Here's the drawing with two shaded views (mm, measured from the low corner). I have some questions. Coordinates: 2 decimals unless noted, no trailing zeros. Order: outer loops, then holes, each group sorted by start corner. A loop starts at its lowest first (then second) coordinate and runs counter-clockwise, first axis right, second up. Notation, with made-up numbers: (-40, 61.5) - (-31, 61.5) arc R16 ccw to (-31, 73.5) - close; hole circle Ø3 at (-16, 20.5). An arc over 180 degrees is marked (long way). One line per item, written item: value. Start each with the question number.
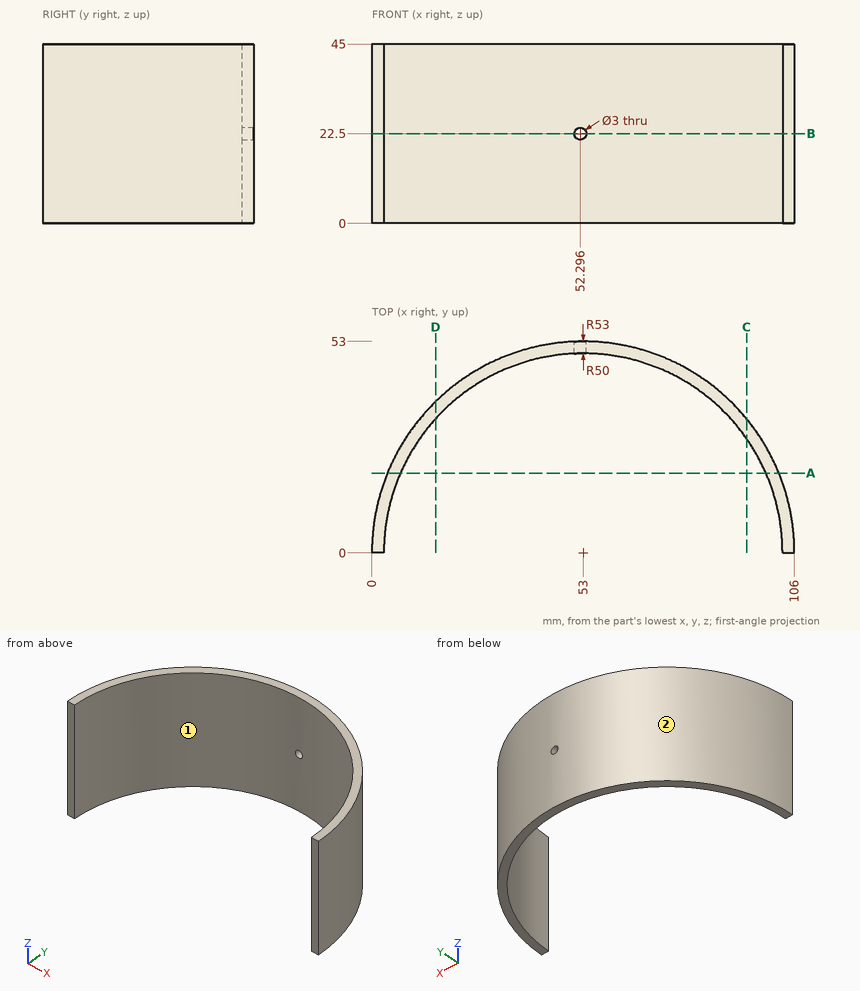
Q1. I want a section at A-A on y = 20. Please give me the cut outline in (x, z) (1 decimal).
Q2. If I drill on L1, parallel to X at y = 21.5, z = 7.5 (1 decimal); L2, parallel to X at y = 9, z = 41; L3, parallel to Y at x = 52, z = 36, over which ranges is the centre line in solid material (lowest first)?
Q3. We'd pull the mould along X, two halves only. Please class the marked faces 1 and 2: +X half, -X half, draft (parallel to the pull), parting line (faces both ways), or undercut.
Q4. I want a section at C-C on x = 94. Please give me the cut outline in (y, z) (1 decimal).
Q5. I'm going to push flat-ended pins straight in: pin 1 (4 mm diameter, centred on x = 29, z = 23.5, fed in from +Y); pin 2 (8 mm diameter, centred on y = 47, z = 37.5, fed in from -X) (1 decimal); pin 3 (4 mm diameter, centred on y = 26, z = 16, fed in from +X) (1 decimal). Where does each tip first touch, or does it pass through?
Q6. I want a section at B-B on z = 22.5. Please give me the cut outline in (x, y) (1 decimal).
Q7. I want a section at D-D on x = 16. Please give me the cut outline in (y, z), then the cut area to 3 significant figures.
Values follow:
1. outline: (3.9, 0) - (7.2, 0) - (7.2, 45) - (3.9, 45) - close; (98.8, 0) - (102.1, 0) - (102.1, 45) - (98.8, 45) - close
2. L1: x = 4.6 to 7.9, 98.1 to 101.4
2. L2: x = 0.77 to 3.82, 102.18 to 105.23
2. L3: y = 49.99 to 52.99
3. face 1: undercut
3. face 2: parting line
4. outline: (28.6, 0) - (33.6, 0) - (33.6, 45) - (28.6, 45) - close
5. pin 1: stops at y = 48.22
5. pin 2: stops at x = 22
5. pin 3: stops at x = 100.3
6. outline: (0, 0) - (3, 0) arc R50 cw to (50.8, 50) - (50.8, 53) arc R53 ccw to start; (53.8, 50) arc R50 cw to (103, 0) - (106, 0) arc R53 ccw to (53.8, 53) - close
7. outline: (33.63, 0) - (37.95, 0) - (37.95, 45) - (33.63, 45) - close
7. area: 194 mm^2
